from build123d import *

# Parameters (mm, degrees)
F0_W     = 160
F0_H     = 80
F1_DEPTH = 40
F2_W     = 144
F2_H     = 64
F3_DEPTH = 30


with BuildPart() as f1:
    # F0 (on Top) → F1 (new body)
    with BuildSketch(Plane.XY):
        with Locations((-11.728724, -20.738534)):
            Rectangle(F0_W, F0_H)
    extrude(amount=F1_DEPTH)

    # F2 (on Top) → F3 (cut)
    with BuildSketch(Plane.XY):
        with Locations((-11.728724, -20.738534)):
            Rectangle(F2_W, F2_H)
    extrude(amount=F3_DEPTH, mode=Mode.SUBTRACT)


solid = f1.part
The listing builds one solid part. Answer for the finished solid, in the listing's coordinates (mm). A direction names the side the tool comes from. Give positions to 0.01 mm unless a question says otherwise; leave off trailing zeros. Loops run counter-clockwise (first coordinate to the right, second up) from the corner with the lowest first, then second, coordinate; pieces in that order, holes last. Notation, with made-up numbers: (2, -37.75) - (50, -37.75) arc R22 ccw to (50, -30.75) - close; hole circle Ø3 at (16, 22). An arc over 180 degrees is marked (long way). Use one line per item in the form item = value.
1. Which of the six approach directions +Z, -Z, +X, -X, +Y, -Y give full straight-line access (tool end or side, diameter ignored) to faces 5 (the face through (68.271, -21, 20)), 6 (the face through (-13, 11.261, 15))?
Calculated:
face_5 = +Z, -Z, +X, +Y, -Y
face_6 = -Z
2. Section A-A on z = 11 is taken. Give the vertices of the cut face in (x, y).
Calculated:
outline = (-91.73, -60.74) - (68.27, -60.74) - (68.27, 19.26) - (-91.73, 19.26) - close; hole (-83.73, -52.74) - (60.27, -52.74) - (60.27, 11.26) - (-83.73, 11.26) - close
3. The mould has two halves that part along Y. Classify faces 1 (the face through (-13, -60.739, 20)), 2 (the face through (-18, -53, 0)), 3 (the face through (-13, 19.261, 20)), 4 (the face through (-13, -52.739, 15)): pulls with the +Y half, pulls with the -Y half, needs draft (parallel to the pull), parting line crosses it, or undercut.
Calculated:
face_1 = pulls with the -Y half
face_2 = needs draft
face_3 = pulls with the +Y half
face_4 = undercut
4. Given pin 1 Ø19 at (x, y) = (24, -31.5) entering from -Z, flat-ended and moving along its own axis, determine where the tip first touches the part or whether it passes through.
Calculated:
pin_1 = 30
5. Section B-B on y = -16.5 is taken. Give the vertices of the cut face in (x, z), then the cut area to 3 significant figures.
Calculated:
outline = (-91.73, 0) - (-83.73, 0) - (-83.73, 30) - (60.27, 30) - (60.27, 0) - (68.27, 0) - (68.27, 40) - (-91.73, 40) - close
area = 2,080 mm^2
6. Section C-C on x = 56 is taken. Give the vertices of the cut face in (y, z).
Calculated:
outline = (-60.74, 0) - (-52.74, 0) - (-52.74, 30) - (11.26, 30) - (11.26, 0) - (19.26, 0) - (19.26, 40) - (-60.74, 40) - close
7. Find the intervals of material crossed by line 1 along Y through (x, z) = (-37, 9.5); line 2 along X through (y, z) = (-45, 11); line 3 along Z through (x, y) = (-63, -18), in increasing order. Write a range as [from, to].
Calculated:
line_1 = [-60.74, -52.74], [11.26, 19.26]
line_2 = [-91.73, -83.73], [60.27, 68.27]
line_3 = [30, 40]
